Geometry check sheet. Reference: the model listing, model coordinates, mm. Face numbers are marked on the shaded views. Coordinates: 2 decimals unless noted, no trailing zeros. Write each loop counter-clockwise with the first axis right and the second up, starting at its lowest first coordinate (ties: lowest second). Pieces come first, ordered by that corner, then holes.
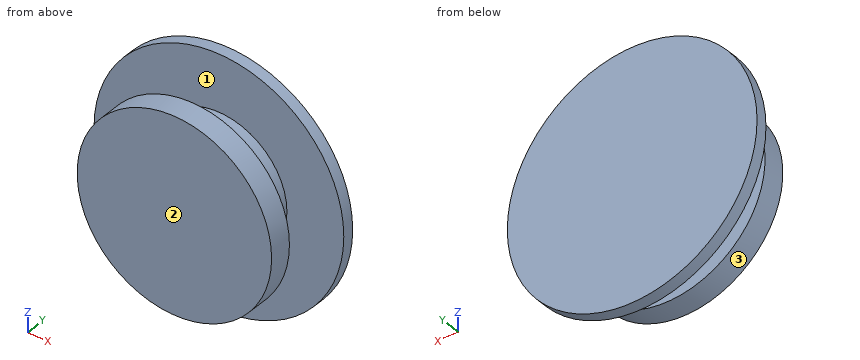
from build123d import *

# Parameters (mm, degrees)
F0_R     = 53.254214
F1_DEPTH = 5
F2_R     = 29.011498
F3_DEPTH = 20
F4_R     = 41.466873
F5_DEPTH = 10


with BuildPart() as f1:
    # F0 (on Front) → F1 (new body)
    with BuildSketch(Plane.XZ):
        Circle(F0_R)
    extrude(amount=F1_DEPTH)

    # F2 (on Front) → F3 (join)
    with BuildSketch(Plane.XZ):
        Circle(F2_R)
    extrude(amount=F3_DEPTH)

    # F4 (on face) → F5 (join)
    with BuildSketch(Plane.XZ.offset(20)):
        Circle(F4_R)
    extrude(amount=F5_DEPTH)


solid = f1.part
1. Sectioned sample at C-C, the plane z = 0. Record the boundary of the cut face in (x, y).
Computed values:
outline: (-53.25, -5) - (-29.01, -5) - (-29.01, -20) - (-41.47, -20) - (-41.47, -30) - (41.47, -30) - (41.47, -20) - (29.01, -20) - (29.01, -5) - (53.25, -5) - (53.25, 0) - (-53.25, 0) - close
2. Draft check along Y on the marked faces 1, 2 and 3. Enter one of: released by +Y, released by -Y, zero draft, split by the parting line, or undercut.
Computed values:
face 1: undercut
face 2: released by -Y
face 3: zero draft
3. Gauge pin test, flat ends, axial feed: pin 1 Ø1 at (x, z) = (-33, 7) entering from +Y; pin 2 Ø1.5 at (x, y) = (6.5, -21) entering from +Z; pin 3 Ø10 at (x, y) = (32, -3.5) entering from +Z; pin 4 Ø6 at (x, y) = (11, -14) entering from +Z. Record the tip position at first contact, or that the pin passes through.
Computed values:
pin 1: stops at y = 0
pin 2: stops at z = 41.07
pin 3: stops at z = 45.9
pin 4: stops at z = 27.89
4. Sectioned sample at A-A, the plane x = -31. Record the boundary of the cut face in (y, z), and give its area (3 significant figures).
Computed values:
outline: (-30, -27.54) - (-20, -27.54) - (-20, 27.54) - (-30, 27.54) - close; (-5, -43.3) - (0, -43.3) - (0, 43.3) - (-5, 43.3) - close
area: 984 mm2
5. Thickness scan on line 1 along Y through (x, z) = (-13, -26.5); line 2 along Y through (x, z) = (-40, -33.5); line 3 along Z through (x, y) = (26.5, -21). Record the ranges inside material, lowest first.
Computed values:
line 1: y = -30 to -20, -5 to 0
line 2: y = -5 to 0
line 3: z = -31.89 to 31.89
6. Sectioned sample at B-B, the plane z = -32. Record the boundary of the cut face in (x, y), and give its area (3 significant figures).
Computed values:
outline: (-42.57, -5) - (42.57, -5) - (42.57, 0) - (-42.57, 0) - close; (-26.37, -30) - (26.37, -30) - (26.37, -20) - (-26.37, -20) - close
area: 953 mm2
7. Sectioned sample at D-D, the plane x = 0. Record the boundary of the cut face in (y, z).
Computed values:
outline: (-30, -41.47) - (-20, -41.47) - (-20, -29.01) - (-5, -29.01) - (-5, -53.25) - (0, -53.25) - (0, 53.25) - (-5, 53.25) - (-5, 29.01) - (-20, 29.01) - (-20, 41.47) - (-30, 41.47) - close
